from build123d import *

# Parameters (mm, degrees)
SKETCH1_W           = 100
SKETCH1_H           = 75
BOSS_EXTRUDE1_DEPTH = 10
FILLET1_R           = 10
SKETCH2_W           = 88.511966946
SKETCH2_H           = 129.218884933
CUT_EXTRUDE1_DEPTH  = 11


with BuildPart() as part:
    # Sketch1 → Boss-Extrude1 (new body)
    with BuildSketch(Plane(origin=(0, 0, 0), x_dir=(1, 0, 0), z_dir=(0, 1, 0))):
        with Locations((50, 37.5)):
            Rectangle(SKETCH1_W, SKETCH1_H)
    extrude(amount=BOSS_EXTRUDE1_DEPTH)

    # Fillet1
    fillet1_edges = [part.edges().sort_by_distance(p)[0] for p in [
        (0, 5, -75),
        (100, 5, -75),
        (100, 5, 0),
        (0, 5, 0),
    ]]
    fillet(fillet1_edges, radius=FILLET1_R)

    # Sketch2 → Cut-Extrude1 (cut, through all)
    with BuildSketch(Plane(origin=(0, 10, 0), x_dir=(1, 0, 0), z_dir=(0, 1, 0))):
        with Locations((14.077953322, 38.537528746)):
            Rectangle(SKETCH2_W, SKETCH2_H)
    extrude(amount=-CUT_EXTRUDE1_DEPTH, mode=Mode.SUBTRACT)


solid = part.part
Could you check a few things on this model? Use its own coordinates, in mm. Give positions to 0.01 mm unless a question says otherwise; leave off trailing zeros. Loops run counter-clockwise (first coordinate to the right, second up) from the corner with the lowest first, then second, coordinate; pieces in that order, holes last. Notation, with made-up numbers: (0, -21) -> (25, -21) arc R18 ccw to (25, -8) -> close; hole circle Ø11 at (20, 42.25). An arc over 180 degrees is marked (long way). Return JSON: item names as keys, results as strings.
Item 1: If we section it at B-B on x = 95.5: List the corners of the cut face in (y, z) for me, plus the area to 3 significant figures.
Geometry results:
{"outline": "(0, -73.35) -> (10, -73.35) -> (10, -1.65) -> (0, -1.65) -> close", "area": "717 mm²"}
Item 2: I need wall thicknesses on L1, parallel to Z at x = 90.5, y = 0.5; L2, parallel to Z at x = 92, y = 9; L3, parallel to X at y = 3, z = -5. Which ranges of each line are inside material? Lowest first, please. Write a range as from..to.
Geometry results:
{"L1": "z = -74.99..-0.01", "L2": "z = -74.8..-0.2", "L3": "x = 58.33..98.66"}
Item 3: I'm going to push a flat-ended pin straight in: pin 1 (1 mm diameter, centred on x = 91, y = 3, fed in from +Z). Where does the tip first touch, or does it pass through?
Geometry results:
{"pin 1": "stops at z = -0.01"}
Item 4: If we section it at A-A on z = -6: List the corners of the cut face in (x, y) for me, plus the area to 3 significant figures.
Geometry results:
{"outline": "(58.33, 0) -> (99.17, 0) -> (99.17, 10) -> (58.33, 10) -> close", "area": "408 mm²"}
